from build123d import *

# Parameters (mm, degrees)
CROQUIS1_R              = 2.5
SALIENTE_EXTRUIR1_DEPTH = 118
CROQUIS2_R              = 1.875
SALIENTE_EXTRUIR2_DEPTH = 2
CROQUIS3_R              = 1.875
SALIENTE_EXTRUIR3_DEPTH = 2


with BuildPart() as part:
    # Croquis1 → Saliente-Extruir1 (new body)
    with BuildSketch(Plane(origin=(0, 0, 0), x_dir=(1, 0, 0), z_dir=(0, 1, 0))):
        Circle(CROQUIS1_R)
    extrude(amount=SALIENTE_EXTRUIR1_DEPTH)

    # Croquis2 → Saliente-Extruir2 (add)
    with BuildSketch(Plane(origin=(0, 118, 0), x_dir=(1, 0, 0), z_dir=(0, 1, 0))):
        Circle(CROQUIS2_R)
    extrude(amount=SALIENTE_EXTRUIR2_DEPTH)

    # Croquis3 → Saliente-Extruir3 (add)
    with BuildSketch(Plane.XZ):
        Circle(CROQUIS3_R)
    extrude(amount=SALIENTE_EXTRUIR3_DEPTH)


solid = part.part
Could you check a few things on this model? Use its own coordinates, in mm. A direction names the side the tool comes from. Coordinates: 2 decimals unless noted, no trailing zeros. Order: outer loops, then holes, each group sorted by start corner. A loop starts at its lowest first (then second) coordinate and runs counter-clockwise, first axis right, second up. Notation, with made-up numbers: (-7.75, 35.5) -> (8.25, 35.5) arc R33 ccw to (8.25, 73.5) -> close; hole circle Ø9 at (83, 59.25). An arc over 180 degrees is marked (long way). One line per item, written item: value. Start each with the question number.
1) Imagine slicing it at C-C on y = 41.5. List the corners of the cut face in (x, z) for me, plus the area to 3 significant figures.
2) Imagine slicing it at A-A on z = 1.1. List the corners of the cut face in (x, y) for me (3 decimals).
3) Imagine slicing it at B-B on x = -1.1. List the corners of the cut face in (y, z) for me (3 decimals), plus the area to 3 significant figures.
4) Which directions (+Z, -Z, +X, -X, +Y, -Y) give clear straight access to the entire face, cutting with the end or side of a thin tool? Please do faces 1 (the flat face through (1, 0, -2)), 2 (the flat face through (0, -2, 0)), 3 (the flat face through (1, 118, -2)).
5) If I drill on L1, parallel to X at y = 7, z = -0.25; L2, parallel to Y at x = 2.1, z = -0.2, over which ranges is the centre line in solid material (lowest first)? Write a range as [from, to].
Answer list:
1. outline: circle Ø5 at (0, 0)
1. area: 19.6 mm2
2. outline: (-2.245, 0) -> (-1.518, 0) -> (-1.518, -2) -> (1.518, -2) -> (1.518, 0) -> (2.245, 0) -> (2.245, 118) -> (1.518, 118) -> (1.518, 120) -> (-1.518, 120) -> (-1.518, 118) -> (-2.245, 118) -> close
3. outline: (-2, -1.518) -> (0, -1.518) -> (0, -2.245) -> (118, -2.245) -> (118, -1.518) -> (120, -1.518) -> (120, 1.518) -> (118, 1.518) -> (118, 2.245) -> (0, 2.245) -> (0, 1.518) -> (-2, 1.518) -> close
3. area: 542 mm2
4. face 1: -Y
4. face 2: +Z, -Z, +X, -X, -Y
4. face 3: +Y
5. L1: x = [-2.49, 2.49]
5. L2: y = [0, 118]
